The listing builds one solid part. Answer for the finished solid, in the listing's coordinates (mm). A direction names the side the tool comes from. Round coordinates to 2 decimals unless told otherwise and drop trailing zeros. Loops run counter-clockwise (first coordinate to the right, second up) from the corner with the lowest first, then second, coordinate; pieces in that order, holes last. Notation, with made-up numbers: (48.25, 67.5) - (54.25, 67.5) arc R26 cw to (54.25, 98.5) - close; hole circle Ø10 at (82.25, 69). An arc over 180 degrees is marked (long way). One line per item, written item: value.
Solid Edge part; units mm, degrees
sketch "Sketch1" plane through (0, 0, 0) normal (0, 0, 1) x (1, 0, 0)
  circle A0 centre (0, 0) radius 9.525
extrude "Protrusion1" add sketch "Sketch1" against normal blind 45.72
sketch "Sketch2" plane through (0, 0, 0) normal (0, 0, 1) x (1, 0, 0)
  line L0 (8.9619, -15.5225) -> (17.9238, 0)
  line L1 (17.9238, 0) -> (8.9619, 15.5225)
  line L2 (8.9619, 15.5225) -> (-8.9619, 15.5225)
  line L3 (-8.9619, 15.5225) -> (-17.9238, 0)
  line L4 (-17.9238, 0) -> (-8.9619, -15.5225)
  line L5 (-8.9619, -15.5225) -> (8.9619, -15.5225)
extrude "ExtrudedProtrusion_2" add sketch "Sketch2" along normal blind 6.35
fillet "Round_1" radius 1.905 6 edges at (13.4429, -7.7612, 6.35) (0, -15.5225, 6.35) (-13.4429, -7.7612, 6.35) (-13.4429, 7.7612, 6.35) (0, 15.5225, 6.35) (13.4429, 7.7612, 6.35)
chamfer "Chamfer_1" distance 1.27 angle 45 1 edges at (-9.525, 0, -45.72)
chamfer "Chamfer_2" distance 0.635 angle 45 6 edges at (-13.4429, -7.7612, 0) (-13.4429, 7.7612, 0) (0, 15.5225, 0) (13.4429, 7.7612, 0) (13.4429, -7.7612, 0) (0, -15.5225, 0)
1) Consider L1, parallel to Z at x = 8, y = 9; L2, parallel to Y at x = 0, z = -3.5 (3 decimals); L3, parallel to Y at x = 2.5, z = -24. Determine where each line is inside the solid, lowest interval first.
Final values:
L1: 0 to 6.35
L2: -9.525 to 9.525
L3: -9.19 to 9.19
2) A cutting plane is placed at B-B on z = -23. Give the vertices of the cut face in (x, y) (3 decimals).
Final values:
outline: circle Ø19.05 at (0, 0)
3) For faces 1 (the cylindrical face through (-12.88, -7.58, 5.81)), 2 (the cylindrical face through (-7.559, -5.796, -21.914)), determine the directions among +Z, -Z, +X, -X, +Y, -Y from which every point of the face is accessible in a straight line to the end or side of a thin tool.
Final values:
face 1: +Z, -X, -Y
face 2: -Z
4) Each of these flat-tipped pins is pushed along its axis until it touches: pin 1 Ø3 at (x, z) = (4, -4.5) entering from -Y; pin 2 Ø6 at (x, z) = (0, -19.5) entering from +Y (3 decimals); pin 3 Ø10 at (y, z) = (5.5, -22) entering from +X. Where does it stop, or does it pass through?
Final values:
pin 1: y = -9.19
pin 2: y = 9.525
pin 3: x = 9.51
